The figure shows three views and two pictorial views of one solid part (mm, origin at its lowest corner). Answer the questions. Coordinates: 2 decimals unless noted, no trailing zeros. Order: outer loops, then holes, each group sorted by start corner. A loop starts at its lowest first (then second) coordinate and runs counter-clockwise, first axis right, second up. Notation, with made-up numbers: (12.5, 80) -> (37.5, 80) arc R16 ccw to (37.5, 93) -> close; hole circle Ø1 at (7, -39). An arc over 180 degrees is marked (long way). Write item = value, one per line.
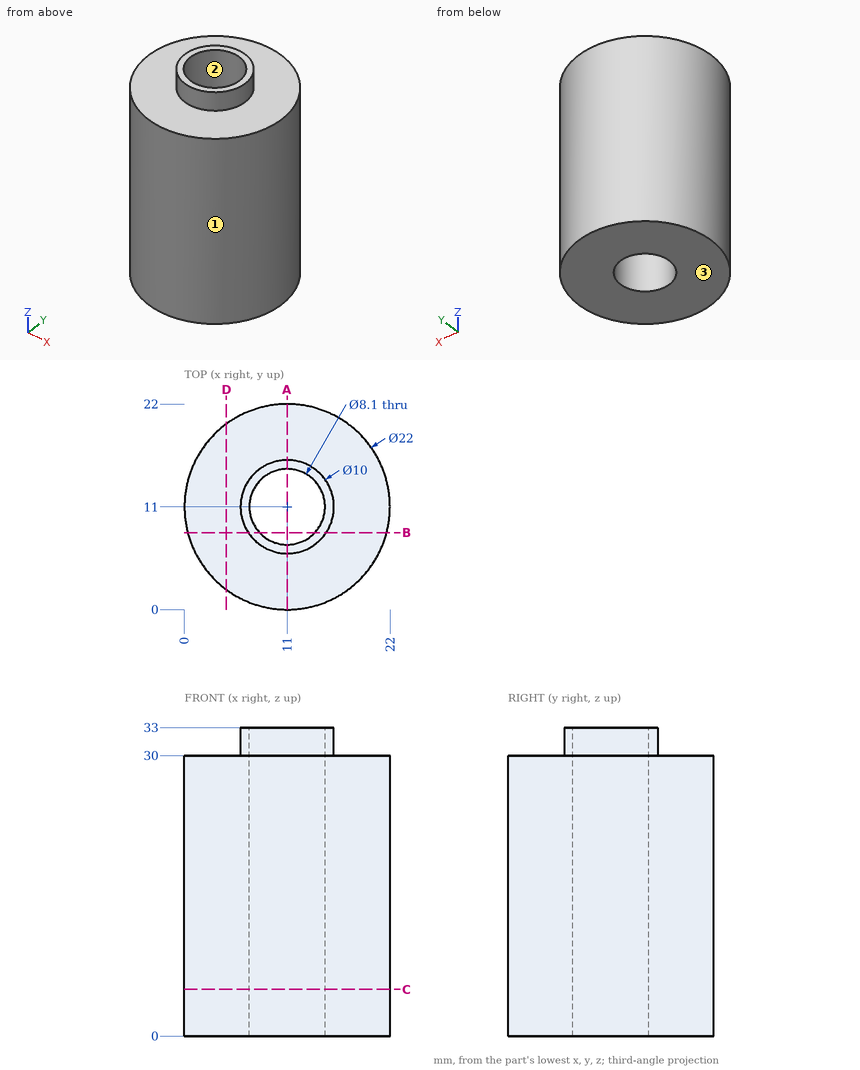
Q1. Section D-D, the plane x = 4.5 is taken. Give the vertices of the cut face in (y, z), plus the area to 3 significant figures.
The answers:
outline = (2.13, 0) -> (19.87, 0) -> (19.87, 30) -> (2.13, 30) -> close
area = 532 mm2
Q2. Section C-C, the plane z = 5 is taken. Give the vertices of the cut face in (x, y), plus the area to 3 significant figures.
The answers:
outline = circle Ø22 at (11, 11); hole circle Ø8.1 at (11, 11)
area = 329 mm2
Q3. Find the intervals of material crossed by line 1 along Y through (x, z) = (11, 11.5); line 2 along Z through (x, y) = (19.25, 15); line 3 along X through (y, z) = (11.25, 19), in increasing order.
The answers:
line_1 = 0 to 6.95, 15.05 to 22
line_2 = 0 to 30
line_3 = 0 to 6.96, 15.04 to 22
Q4. Section B-B, the plane y = 8.25 is taken. Give the vertices of the cut face in (x, z).
The answers:
outline = (0.35, 0) -> (8.03, 0) -> (8.03, 33) -> (6.82, 33) -> (6.82, 30) -> (0.35, 30) -> close; (13.97, 0) -> (21.65, 0) -> (21.65, 30) -> (15.18, 30) -> (15.18, 33) -> (13.97, 33) -> close
Q5. The mould has two halves that part along X. Classify the marked faces 1, 2 and 3: released by +X, released by -X, zero draft, split by the parting line, or undercut.
The answers:
face_1 = split by the parting line
face_2 = undercut
face_3 = zero draft
Q6. Each of these flat-tipped pins is pushed along its axis until it touches: pin 1 Ø6 at (y, z) = (15, 7.5) entering from -X; pin 2 Ø2 at (x, z) = (19, 22) entering from -Y; pin 3 Ø4 at (y, z) = (19, 4) entering from -X. Where does it stop, or does it pass through?
The answers:
pin_1 = 0.05
pin_2 = 2.51
pin_3 = 1.78
Q7. Section A-A, the plane x = 11 is taken. Give the vertices of the cut face in (y, z).
The answers:
outline = (0, 0) -> (6.95, 0) -> (6.95, 33) -> (6, 33) -> (6, 30) -> (0, 30) -> close; (15.05, 0) -> (22, 0) -> (22, 30) -> (16, 30) -> (16, 33) -> (15.05, 33) -> close
